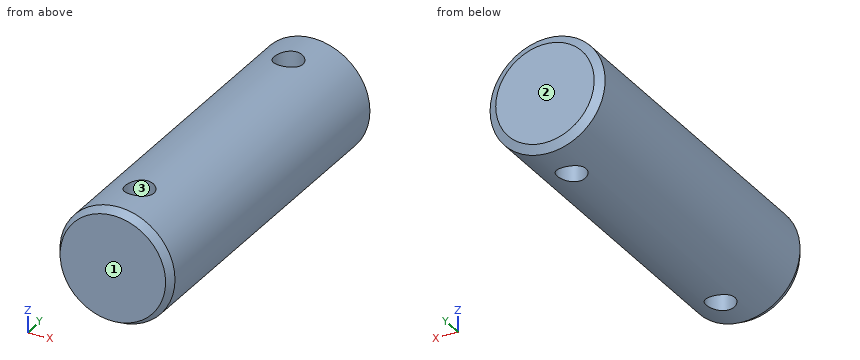
from build123d import *

# Parameters (mm, degrees)
SKETCH1_R               = 6
BOSS_EXTRUDE1_DEPTH     = 19
CHAMFER1_SIZE           = 0.5
CHAMFER1_SIZE2          = 0.866025404
CHAMFER1_PART_2_SIZE    = 0.5
CHAMFER1_PART_2_SIZE2   = 0.866025404
SKETCH2_R               = 1.5
CUT_EXTRUDE1_DEPTH      = 7
CUT_EXTRUDE1_DEPTH_BACK = 7


with BuildPart() as part:
    # Sketch1 → Boss-Extrude1 (new body, symmetric)
    with BuildSketch(Plane(origin=(0, 0, 0), x_dir=(1, 0, 0), z_dir=(0, 1, 0))):
        Circle(SKETCH1_R)
    extrude(amount=BOSS_EXTRUDE1_DEPTH, both=True)

    # Chamfer1
    chamfer1_edges = [part.edges().sort_by_distance(p)[0] for p in [
        (-6, -19, 0),
    ]]
    chamfer1_side = [part.faces().sort_by_distance(p)[0] for p in [
        (0, -19, 0),
    ]]
    chamfer(chamfer1_edges, length=CHAMFER1_SIZE, length2=CHAMFER1_SIZE2, reference=chamfer1_side[0])

    # Chamfer1 part 2
    chamfer1_part_2_edges = [part.edges().sort_by_distance(p)[0] for p in [
        (-6, 19, 0),
    ]]
    chamfer1_part_2_side = [part.faces().sort_by_distance(p)[0] for p in [
        (-6, 0, 0),
    ]]
    chamfer(chamfer1_part_2_edges, length=CHAMFER1_PART_2_SIZE, length2=CHAMFER1_PART_2_SIZE2, reference=chamfer1_part_2_side[0])

    # Sketch2 → Cut-Extrude1 (cut, two sides)
    with BuildSketch(Plane.XY) as cut_extrude1_sk:
        with Locations((0, 14)):
            Circle(SKETCH2_R)
        with Locations((0, -14)):
            Circle(SKETCH2_R)
    extrude(amount=CUT_EXTRUDE1_DEPTH, mode=Mode.SUBTRACT)
    extrude(cut_extrude1_sk.sketch, amount=-CUT_EXTRUDE1_DEPTH_BACK, mode=Mode.SUBTRACT)


solid = part.part
Check sheet for the modelled part. Datum: model origin and axes. Units: mm. Face numbers are marked on the shaded views. Round coordinates to 2 decimals unless told otherwise and drop trailing zeros. Order: outer loops, then holes, each group sorted by start corner. A loop starts at its lowest first (then second) coordinate and runs counter-clockwise, first axis right, second up.
(1) Scan lines: probe 1 along Y at (x, z) = (0, -0.75); probe 2 along X at (y, z) = (14, 0); probe 3 along X at (y, z) = (14.5, 0.5). Record each from-to range of solid material in increasing order.
(2) Go/stop test with flat-tipped pins: P1, Ø2, axis at x = 4.5, y = 2.5, coming from the -Z side; P2, Ø5, axis at y = 14, z = -4.5, coming from the -X side; P3, Ø4, axis at y = -1.5, z = -2.5, coming from the +X side. Record where each tip stops, or that it passes through.
(3) Cross-section at D-D, the plane y = -14. Enter the section's corners in (x, z).
(4) Cross-section at A-A, the plane x = 0. Enter the section's corners in (y, z), and give its area (3 significant figures).
(5) Cross-section at C-C, the plane y = 1.5. Enter the section's corners in (x, z), and give its area (3 significant figures).
(6) Cross-section at B-B, the plane z = 0. Enter the section's corners in (x, y).
(7) Draft check along Y on the marked faces 1, 2 and 3. Enter one of: pulls with the +Y half, pulls with the -Y half, needs draft (parallel to the pull), parting line crosses it, or undercut.
Check sheet entries:
1. probe 1: y = -19 to -15.5, -12.5 to 12.5, 15.5 to 19
1. probe 2: x = -6 to -1.5, 1.5 to 6
1. probe 3: x = -5.98 to -1.41, 1.41 to 5.98
2. P1: stops at z = -4.87
2. P2: stops at x = -5.66
2. P3: stops at x = 5.98
3. outline: (-1.5, -5.81) - (-1.5, 5.81) arc R6 ccw to start; (1.5, -5.81) arc R6 ccw to (1.5, 5.81) - close
4. outline: (-19, -5.5) - (-18.13, -6) - (-15.5, -6) - (-15.5, 6) - (-18.13, 6) - (-19, 5.5) - close; (-12.5, -6) - (12.5, -6) - (12.5, 6) - (-12.5, 6) - close; (15.5, -6) - (18.5, -6) - (19, -5.13) - (19, 5.13) - (18.5, 6) - (15.5, 6) - close
4. area: 383 mm2
5. outline: circle Ø12 at (0, 0)
5. area: 113 mm2
6. outline: (-6, -18.13) - (-5.5, -19) - (5.5, -19) - (6, -18.13) - (6, 18.5) - (5.13, 19) - (-5.13, 19) - (-6, 18.5) - close; hole circle Ø3 at (0, -14); hole circle Ø3 at (0, 14)
7. face 1: pulls with the -Y half
7. face 2: pulls with the +Y half
7. face 3: undercut
